from build123d import *

# Parameters (mm, degrees)
SKETCH_1_W          = 63
SKETCH_1_H          = 20
EXTRUDE_1_DEPTH     = 3
HOLE_WIZARD_M5_1_D  = 5.5
CUT_EXTRUDE_1_DEPTH = 34.185087012
CHAMFER_1_SIZE      = 7


with BuildPart() as part:
    # 草图1 → 凸台-拉伸1 (new body)
    with BuildSketch(Plane.XY):
        Rectangle(SKETCH_1_W, SKETCH_1_H)
    extrude(amount=EXTRUDE_1_DEPTH)

    # M5 间隙孔1 (through all)
    with Locations(Plane(origin=(0, 0, 0), x_dir=(-1, 0, 0), z_dir=(0, 0, -1))):
        with Locations((25.5, 5), (-4.5, 5)):
            Hole(HOLE_WIZARD_M5_1_D / 2)

    # 草图5 → 切除-拉伸1 (cut, through all)
    with BuildSketch(Plane(origin=(0, 0, 0), x_dir=(-1, 0, 0), z_dir=(0, 0, -1))):
        with BuildLine():
            Line((-23.5, 3.5), (-31.5, 3.5))
            Line((-31.5, 3.5), (-31.5, -3.5))
            Line((-31.5, -3.5), (-23.5, -3.5))
            ThreePointArc((-23.5, -3.5), (-20, 0), (-23.5, 3.5))
        make_face()
    extrude(amount=-CUT_EXTRUDE_1_DEPTH, mode=Mode.SUBTRACT)

    # 倒角1
    chamfer_1_edges = [part.edges().sort_by_distance(p)[0] for p in [
        (-31.5, -10, 1.5),
    ]]
    chamfer(chamfer_1_edges, length=CHAMFER_1_SIZE)


solid = part.part
The listing builds one solid part. Answer for the finished solid, in the listing's coordinates (mm). A direction names the side the tool comes from. Round coordinates to 2 decimals unless told otherwise and drop trailing zeros. Write each loop counter-clockwise with the first axis right and the second up, starting at its lowest first coordinate (ties: lowest second). Pieces come first, ordered by that corner, then holes. Notation, with made-up numbers: M 13,5.5 L 39,5.5 A19 cw 39,28.5 Z; hole C 62.25,60.5 d2. An arc over 180 degrees is marked long. Write each question's results on one line, items separated by ' | '. Start each with the question number.
(1) The part is cut by section B-B, the plane z = 0.75. Write down the section's boundary in (x, y), and give its area (3 significant figures).
(2) This flat-tipped pin is pushed along its axis until it touches: P1, Ø1.5, axis at y = 0.5, z = 1, coming from the +X side. Where does it stop, or does it pass through?
(3) The part is cut by section C-C, the plane x = 4.5. Write down the section's boundary in (y, z).
(4) Find the intervals of material crossed by line 1 (Y direction, x = 4.5, z = 2.35); line 2 (X direction, y = 6.75, z = 1.35); line 3 (Y direction, x = 26, z = 0.9), in increasing order.
(5) For faces 5 (the flat face through (27, 3.5, 1)), 6 (the flat face through (-28, -6.5, 1.5)), determine the directions among +Z, -Z, +X, -X, +Y, -Y from which every point of the face is accessible in a straight line to the end or side of a thin tool.
(6) The part is cut by section A-A, the plane y = 5. Write down the section's boundary in (x, z), and give its area (3 significant figures).
(7) The part is cut by section D-D, the plane x = -25.5. Write down the section's boundary in (y, z), and give its area (3 significant figures).
(8) Determine the mould class of faces 1 (the cylindrical face through (5.77, 2.56, 1.52)), 2 (the flat face through (28, -3.5, 1)), 3 (the flat face through (31.5, 7, 1)), 4 (the cylindrical face through (-28.247, 5.121, 1.521)) for opening direction X: +X half, -X half, draft (parallel to the pull), parting line (faces both ways), or undercut.
Worked answers:
1) outline: M -31.5,-3 L -24.5,-10 L 31.5,-10 L 31.5,-3.5 L 23.5,-3.5 A3.5 cw 23.5,3.5 L 31.5,3.5 L 31.5,10 L -31.5,10 Z; hole C -25.5,5 d5.5; hole C 4.5,5 d5.5 | area: 1,110 mm²
2) P1: stops at x = 20.23
3) outline: M -10,0 L 2.25,0 L 2.25,3 L -10,3 Z; M 7.75,0 L 10,0 L 10,3 L 7.75,3 Z
4) line 1: y = -10 to 2.25, 7.75 to 10 | line 2: x = -31.5 to -27.62, -23.38 to 2.38, 6.62 to 31.5 | line 3: y = -10 to -3.5, 3.5 to 10
5) face 5: +Z, -Z, +X | face 6: +Z, -Z, -X, -Y
6) outline: M -31.5,0 L -28.25,0 L -28.25,3 L -31.5,3 Z; M -22.75,0 L 1.75,0 L 1.75,3 L -22.75,3 Z; M 7.25,0 L 31.5,0 L 31.5,3 L 7.25,3 Z | area: 156 mm²
7) outline: M -9,0 L 2.25,0 L 2.25,3 L -9,3 Z; M 7.75,0 L 10,0 L 10,3 L 7.75,3 Z | area: 40.5 mm²
8) face 1: undercut | face 2: draft | face 3: +X half | face 4: undercut
